from build123d import *

# Parameters (mm, degrees)
F0_W     = 780
F0_H     = 430
F1_DEPTH = 8
F3_W     = 350
F3_H     = 330
F4_DEPTH = 25
F5_W     = 360
F5_H     = 340
F5_W_2   = 350
F5_H_2   = 330
F6_DEPTH = 150
F7_W     = 360
F7_H     = 340
F7_W_2   = 350
F7_H_2   = 330
F8_DEPTH = 5
F9_R     = 30
F10_R    = 5


with BuildPart() as f1:
    # F0 (on Top) → F1 (new body)
    with BuildSketch(Plane.XY):
        Rectangle(F0_W, F0_H)
    extrude(amount=F1_DEPTH)

    # F3 (on face) → F4 (cut)
    with BuildSketch(Plane.XY.offset(8)):
        with Locations((-175, 0)):
            Rectangle(F3_W, F3_H)
    extrude(amount=-F4_DEPTH, mode=Mode.SUBTRACT)

    # F5 (on face) → F6 (join)
    with BuildSketch(Plane(origin=(0, 0, 0), x_dir=(1, 0, 0), z_dir=(0, 0, -1))):
        with Locations((-175, 0)):
            Rectangle(F5_W, F5_H)
        with Locations((-175, 0)):
            Rectangle(F5_W_2, F5_H_2, mode=Mode.SUBTRACT)
    extrude(amount=F6_DEPTH)

    # F7 (on face) → F8 (join)
    with BuildSketch(Plane(origin=(0, 0, -150), x_dir=(1, 0, 0), z_dir=(0, 0, -1))):
        with Locations((-175, 0)):
            Rectangle(F7_W, F7_H)
        with Locations((-175, 0)):
            Rectangle(F7_W_2, F7_H_2, mode=Mode.SUBTRACT)
        with Locations((-175, 0)):
            Rectangle(F7_W_2, F7_H_2)
    extrude(amount=F8_DEPTH)

    # F9
    f9_edges = [f1.edges().sort_by_distance(p)[0] for p in [
        (-175, 165, -150),
        (0, 0, -150),
        (-175, -165, -150),
        (0, -165, -71),
        (0, 165, -71),
        (-350, 165, -71),
        (-350, 0, -150),
        (-350, -165, -71),
    ]]
    fillet(f9_edges, radius=F9_R)

    # F10
    f10_edges = [f1.edges().sort_by_distance(p)[0] for p in [
        (-390, 0, 8),
        (-175, -165, 8),
        (-341.213203, -156.213203, 8),
        (-8.786797, -156.213203, 8),
        (-350, 0, 8),
        (0, 0, 8),
        (-341.213203, 156.213203, 8),
        (-8.786797, 156.213203, 8),
        (-175, 165, 8),
        (390, 0, 8),
        (0, -215, 8),
        (0, 215, 8),
    ]]
    fillet(f10_edges, radius=F10_R)


solid = f1.part
The listing builds one solid part. Answer for the finished solid, in the listing's coordinates (mm). A direction names the side the tool comes from. Give positions to 0.01 mm unless a question says otherwise; leave off trailing zeros. Order: outer loops, then holes, each group sorted by start corner. A loop starts at its lowest first (then second) coordinate and runs counter-clockwise, first axis right, second up. Notation, with made-up numbers: (-30.5, -24) - (-26.5, -24) arc R6 cw to (-26.5, -18) - close; hole circle Ø7 at (-30.75, -36.75). An arc over 180 degrees is marked (long way). One line per item, written item: value. Start each with the question number.
1) A tool of negligible diameter and unlimited length cuts with its end or side. For faces 4 (the face through (5, 2, -76)), 5 (the face through (-172.97, 155.979, -141.445)), 6 (the face through (-178, -170, -76)), 7 (the face through (-355, 2, -76)), from which of +Z, -Z, +X, -X, +Y, -Y can it reach the whole face along a straight path? Write none if from no direction.
2) A cutting plane is placed at A-A on z = -55. Give the vertices of the cut face in (x, y), then the cut area to 3 significant figures.
3) The mould has two halves that part along Y. Classify faces 1 (the face through (-178, -2, -155)), 2 (the face through (-177, 165, -58)), 3 (the face through (-178, 170, -76)): released by +Y, released by -Y, zero draft, split by the parting line, or undercut.
4) Given pin 1 Ø8 at (x, z) = (-285, -126) entering from +Y; pin 2 Ø4 at (y, z) = (86, -61) entering from -X; pin 3 Ø2 at (x, y) = (-294.5, 120.5) entering from +Z, each flat-ended and moving along its own axis, determine where each tip first touches the part or whether it passes through.
5) Find the intervals of material crossed by L1, parallel to X at y = 60.5, z = -100.5; L2, parallel to Y at x = -207.5, z = -79; L3, parallel to Z at x = -47.5, y = 59, in increasing order.
6) A cutting plane is placed at B-B on y = 18. Give the vertices of the cut face in (x, z), then the cut area to 3 significant figures.
7) A cutting plane is placed at C-C on x = -247. Give the vertices of the cut face in (y, z).
8) A cutting plane is placed at D-D on x = 70.5. Give the vertices of the cut face in (y, z).
Answer sheet:
1. face 4: -Z, +X, +Y, -Y
1. face 5: +Z
1. face 6: -Z, +X, -X, -Y
1. face 7: -Z, -X, +Y, -Y
2. outline: (-355, -170) - (5, -170) - (5, 170) - (-355, 170) - close; hole (-350, -135) arc R30 ccw to (-320, -165) - (-30, -165) arc R30 ccw to (0, -135) - (0, 135) arc R30 ccw to (-30, 165) - (-320, 165) arc R30 ccw to (-350, 135) - close
2. area: 7,670 mm2
3. face 1: zero draft
3. face 2: undercut
3. face 3: released by +Y
4. pin 1: stops at y = 170
4. pin 2: stops at x = -355
4. pin 3: stops at z = -150
5. L1: x = -355 to -350, 0 to 5
5. L2: y = -170 to -165, 165 to 170
5. L3: z = -155 to -150
6. outline: (-390, 0) - (-355, 0) - (-355, -155) - (5, -155) - (5, 0) - (390, 0) - (390, 3) arc R5 ccw to (385, 8) - (5, 8) arc R5 ccw to (0, 3) - (0, -120) arc R30 cw to (-30, -150) - (-320, -150) arc R30 cw to (-350, -120) - (-350, 3) arc R5 ccw to (-355, 8) - (-385, 8) arc R5 ccw to (-390, 3) - close
6. area: 7,100 mm2
7. outline: (-215, 0) - (-170, 0) - (-170, -155) - (170, -155) - (170, 0) - (215, 0) - (215, 3) arc R5 ccw to (210, 8) - (170, 8) arc R5 ccw to (165, 3) - (165, -120) arc R30 cw to (135, -150) - (-135, -150) arc R30 cw to (-165, -120) - (-165, 3) arc R5 ccw to (-170, 8) - (-210, 8) arc R5 ccw to (-215, 3) - close
8. outline: (-215, 0) - (215, 0) - (215, 3) arc R5 ccw to (210, 8) - (-210, 8) arc R5 ccw to (-215, 3) - close
